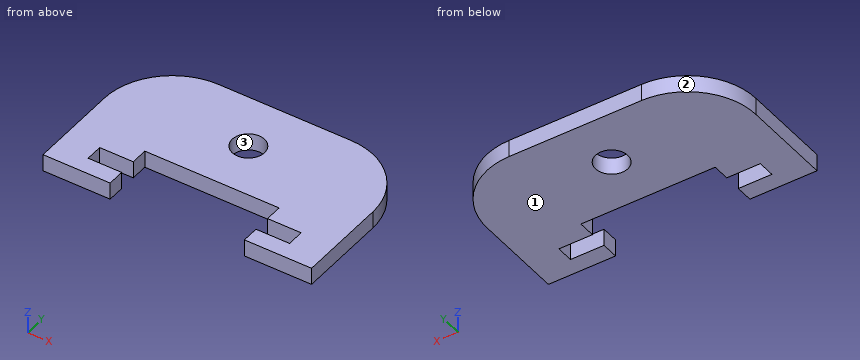
```python
from build123d import *

# Parameters (mm, degrees)
BOSS_EXTRUDE1_DEPTH     = 6.35
CUT_EXTRUDE1_DEPTH      = 108.890326167
CUT_EXTRUDE1_DEPTH_BACK = 108.890326167
SKETCH2_R               = 5.999999938
FILLET1_R               = 25.4
CUT_EXTRUDE2_DEPTH      = 108.890326167
CUT_EXTRUDE2_DEPTH_BACK = 108.890326167
SKETCH3_W               = 12.499999987
SKETCH3_H               = 6.35


with BuildPart() as part:
    # Sketch1 → Boss-Extrude1 (new body)
    with BuildSketch(Plane.XY):
        Polygon((24.999999974, 0), (74.999999924, 0), (74.999999923, -6.35), (74.999999923, -19.05), (99.999999898, -19.05), (99.999999898, -6.35), (99.999999898, 0), (99.999999898, 40.00000001), (0, 40.00000001), (0, 0), (0, -6.35), (0, -19.05), (24.999999974, -19.05), (24.999999974, -6.35), align=None)
    extrude(amount=BOSS_EXTRUDE1_DEPTH)

    # Sketch2 → Cut-Extrude1 (cut, two sides: drawn at the far end of the back side and taken through both)
    with BuildSketch(Plane.XY.offset(6.35).offset(-CUT_EXTRUDE1_DEPTH_BACK)):
        with Locations((49.999999949, 20.000000005)):
            Circle(SKETCH2_R)
    extrude(amount=CUT_EXTRUDE1_DEPTH + CUT_EXTRUDE1_DEPTH_BACK, mode=Mode.SUBTRACT)

    # Fillet1
    fillet1_edges = [part.edges().sort_by_distance(p)[0] for p in [
        (0, 40.00000001, 3.175),
        (99.999999898, 40.00000001, 3.175),
    ]]
    fillet(fillet1_edges, radius=FILLET1_R)

    # Sketch3 → Cut-Extrude2 (cut, two sides: drawn at the far end of the back side and taken through both)
    with BuildSketch(Plane.XY.offset(6.35).offset(-CUT_EXTRUDE2_DEPTH_BACK)):
        with Locations((81.249999918, -9.525)):
            Rectangle(SKETCH3_W, SKETCH3_H)
        with Locations((18.749999981, -9.525)):
            Rectangle(SKETCH3_W, SKETCH3_H)
    extrude(amount=CUT_EXTRUDE2_DEPTH + CUT_EXTRUDE2_DEPTH_BACK, mode=Mode.SUBTRACT)


solid = part.part
```
Model file for the job. Use its own axes, mm. Face numbers are marked on the shaded views. Coordinates: 2 decimals unless noted, no trailing zeros. Order: outer loops, then holes, each group sorted by start corner. A loop starts at its lowest first (then second) coordinate and runs counter-clockwise, first axis right, second up. Notation, with made-up numbers: M 62,-22.5 L 73,-22.5 A23 cw 73,-6.5 Z; hole C -28.5,-31.75 d1. An arc over 180 degrees is marked long. Answer as CSV lines item,"result".
(1) Band-saw the part on A-A, the plane y = -1. List the corners of the cut face in (x, z), then the cut area to 4 significant figures.
Geometry says:
outline,"M 0,0 L 25,0 L 25,6.35 L 0,6.35 Z; M 75,0 L 100,0 L 100,6.35 L 75,6.35 Z"
area,"317.5 mm2"
(2) Band-saw the part on C-C, the plane z = 1.5. List the corners of the cut face in (x, y), then the cut area to 3 significant figures.
Geometry says:
outline,"M 0,-19.05 L 25,-19.05 L 25,-12.7 L 12.5,-12.7 L 12.5,-6.35 L 25,-6.35 L 25,0 L 75,0 L 75,-6.35 L 87.5,-6.35 L 87.5,-12.7 L 75,-12.7 L 75,-19.05 L 100,-19.05 L 100,14.6 A25.4 ccw 74.6,40 L 25.4,40 A25.4 ccw 0,14.6 Z; hole C 50,20 d12"
area,"4,400 mm2"
(3) Flat gauge pins, fed straight in: pin 1 (9.5 mm diameter, centred on x = 50, y = 20, fed in from -Z); pin 2 (3 mm diameter, centred on x = 34.5, z = 4.5, fed in from -Y); pin 3 (3 mm diameter, centred on y = 28, z = 2, fed in from -X); pin 4 (2 mm diameter, centred on x = 89, z = 1.5, fed in from +Y). Where does each tip first touch, or does it go through?
Geometry says:
pin 1,"passes through"
pin 2,"stops at y = 0"
pin 3,"stops at x = 2.96"
pin 4,"stops at y = 36.18"
(4) Band-saw the part on D-D, the plane x = 29. List the corners of the cut face in (y, z).
Geometry says:
outline,"M 0,0 L 40,0 L 40,6.35 L 0,6.35 Z"
(5) Pull direction Y, two halves, no side cores. Call the marked faces 1, 2 and 3: +Y half, -Y half, draft (parallel to the pull), parting line (faces both ways), or undercut.
Geometry says:
face 1,"draft"
face 2,"+Y half"
face 3,"undercut"
(6) Band-saw the part on B-B, the plane x = 50. List the corners of the cut face in (y, z), then the cut area to 3 significant figures.
Geometry says:
outline,"M 0,0 L 14,0 L 14,6.35 L 0,6.35 Z; M 26,0 L 40,0 L 40,6.35 L 26,6.35 Z"
area,"178 mm2"
(7) Wall check: line 1 along Y through (x, z) = (50, 4.25); line 2 along Y through (x, z) = (57.5, 3); line 3 along Y through (x, z) = (78, 2.75). Give the ranges that are in metal, low to high.
Geometry says:
line 1,"y = 0 to 14, 26 to 40"
line 2,"y = 0 to 40"
line 3,"y = -19.05 to -12.7, -6.35 to 39.77"
